```python
from build123d import *

# Parameters (mm, degrees)
F0_R     = 45.372538
F1_DEPTH = 25.4
F3_D     = 25.4
F5_D     = 25.4
F6_W     = 56.968233
F6_H     = 8.121184
F7_DEPTH = 25.4


with BuildPart() as f1:
    # F0 (on Front) → F1 (new body)
    with BuildSketch(Plane.XZ):
        with Locations((-15.429733, 7.751094)):
            Circle(F0_R)
    extrude(amount=F1_DEPTH)

    # F3 (through all)
    with Locations(Plane.XZ.offset(25.4)):
        with Locations((-36.322083, 21.740559)):
            Hole(F3_D / 2)

    # F5 (through all)
    with Locations(Plane.XZ.offset(25.4)):
        with Locations((2.110902, 25.776088)):
            Hole(F5_D / 2)

    # F6 (on face) → F7 (join)
    with BuildSketch(Plane.XZ.offset(25.4)):
        with Locations((-16.729575, -9.404827)):
            Rectangle(F6_W, F6_H)
    extrude(amount=F7_DEPTH)


solid = f1.part
```
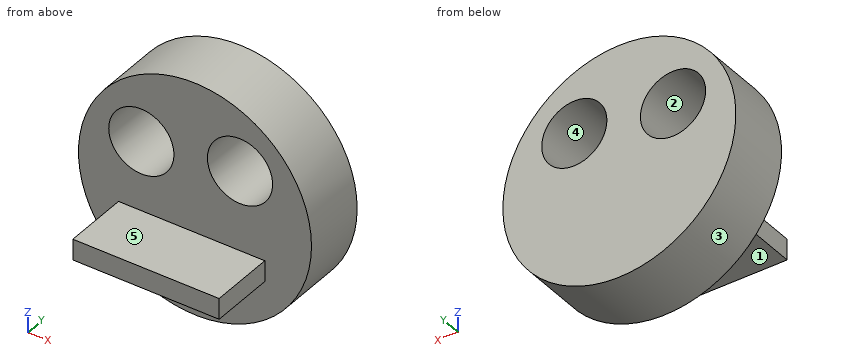
Input: part model. Units: mm. Frame: model coordinates. Face numbers are marked on the shaded views. A direction names the side the tool comes from. Round coordinates to 2 decimals unless told otherwise and drop trailing zeros. Order: outer loops, then holes, each group sorted by start corner. A loop starts at its lowest first (then second) coordinate and runs counter-clockwise, first axis right, second up. Notation, with made-up numbers: (58.5, -23.75) - (108.5, -23.75) arc R19 ccw to (108.5, 8.25) - close; hole circle Ø4 at (81.25, -25.5). An arc over 180 degrees is marked (long way). Answer in a Markdown table with one row per item.
Item 1: Section query C-C (y = -41). Return the cut outline in (x, z).
Model answer:
| item | result |
|---|---|
| outline | (-45.21, -13.47) - (11.75, -13.47) - (11.75, -5.34) - (-45.21, -5.34) - close |
Item 2: Section query D-D (x = 5.5). Return the cut outline in (y, z), then the cut area to 3 significant figures.
Model answer:
| item | result |
|---|---|
| outline | (-50.8, -13.47) - (-25.4, -13.47) - (-25.4, -32.51) - (0, -32.51) - (0, 13.54) - (-25.4, 13.54) - (-25.4, -5.34) - (-50.8, -5.34) - close; (-25.4, 38.02) - (0, 38.02) - (0, 48.01) - (-25.4, 48.01) - close |
| area | 1,630 mm² |
Item 3: Mould query, pull axis Z, two halves, no side actions, for the marked faces 1, 2 and 3. Classes: released by +Z, released by -Z, zero draft, split by the parting line, or undercut.
Model answer:
| item | result |
|---|---|
| face 1 | released by -Z |
| face 2 | undercut |
| face 3 | split by the parting line |
Item 4: Reachability of the marked faces 4 and 5 from +Z, -Z, +X, -X, +Y, -Y: full face, straight path, thin tool, end or side. Return the list, or none.
Model answer:
| item | result |
|---|---|
| face 4 | +Y, -Y |
| face 5 | +Z, +X, -X, -Y |
Item 5: Section query A-A (x = -35). Return the cut outline in (y, z).
Model answer:
| item | result |
|---|---|
| outline | (-50.8, -13.47) - (-25.4, -13.47) - (-25.4, -33.18) - (0, -33.18) - (0, 9.11) - (-25.4, 9.11) - (-25.4, -5.34) - (-50.8, -5.34) - close; (-25.4, 34.37) - (0, 34.37) - (0, 48.69) - (-25.4, 48.69) - close |
Item 6: Pin query (flat end, axial travel): pin 1 (12.5 mm diameter, centred on x = -28.5, y = -37, fed in from -Z); pin 2 (7.5 mm diameter, centred on x = -15.5, y = -35.5, fed in from +Z); pin 3 (6 mm diameter, centred on x = -11, z = 38.5, fed in from -Y). Return the tip coordinate at first contact, or that it passes through.
Model answer:
| item | result |
|---|---|
| pin 1 | stops at z = -13.47 |
| pin 2 | stops at z = -5.34 |
| pin 3 | stops at y = -25.4 |
Item 7: Section query B-B (z = -7.5). Return the cut outline in (x, y).
Model answer:
| item | result |
|---|---|
| outline | (-58.16, -25.4) - (-45.21, -25.4) - (-45.21, -50.8) - (11.75, -50.8) - (11.75, -25.4) - (27.3, -25.4) - (27.3, 0) - (-58.16, 0) - close |
Item 8: Line query: line 1 (Y direction, x = -18, z = 43); line 2 (X direction, y = -27, z = -6.5); line 3 (Z direction, x = -35, y = -29). Output: solid intervals per line, ascending.
Model answer:
| item | result |
|---|---|
| line 1 | y = -25.4 to 0 |
| line 2 | x = -45.21 to 11.75 |
| line 3 | z = -13.47 to -5.34 |
